Work out the finished part from the listing and answer in its coordinate system (mm). Coordinates: 2 decimals unless noted, no trailing zeros. Write each loop counter-clockwise with the first axis right and the second up, starting at its lowest first coordinate (ties: lowest second). Pieces come first, ordered by that corner, then holes. Notation, with made-up numbers: (39.5, 53.25) - (93.5, 53.25) arc R13 ccw to (93.5, 68.25) - close; hole circle Ø6 at (-7.75, -2). An arc over 180 degrees is marked (long way). One line per item, written item: value.
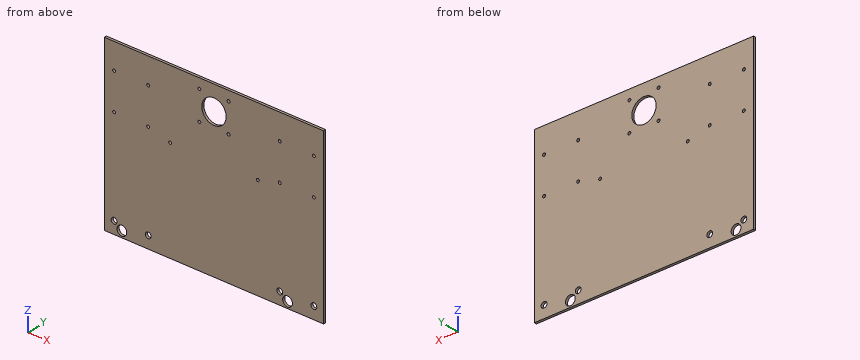
Autodesk Inventor part; units mm, degrees
ref_plane "YZ Plane" through (0, 0, 0) normal (1, 0, 0) x (0, 1, 0)
ref_plane "XZ Plane" through (0, 0, 0) normal (0, 1, 0) x (-1, 0, 0)
ref_plane "XY Plane" through (0, 0, 0) normal (0, 0, 1) x (1, 0, 0)
sketch "Sketch1" plane through (0, 0, 0) normal (0, 1, 0) x (-1, 0, 0)
  line L0 (225, 175) -> (-225, 175)
  line L1 (-225, 175) -> (-225, -175)
  line L2 (-225, -175) -> (225, -175)
  line L3 (225, -175) -> (225, 175)
  line L4 (225, 175) -> (-225, -175) construction
  line L5 (-225, 175) -> (225, -175) construction
  point P0 (0, 0)
  dimension "d0" = 450
  dimension "d1" = 350
extrude "Extrusion1" add sketch "Sketch1" along normal blind 5
sketch "Sketch2" plane through (0, 0, 0) normal (0, -1, 0) x (1, 0, 0)
  line L0 (225, 175) -> (225, -175)
  line L1 (-225, 175) -> (225, 175)
  line L2 (-225, -175) -> (-225, 175)
  line L3 (225, -175) -> (-225, -175)
  line L4 (-198.5, -164) -> (-198.5, -170)
  line L5 (-220, -170) -> (-198.5, -170)
  line L6 (-220, -115) -> (-220, -170)
  line L7 (-220, -115) -> (-120, -115)
  line L8 (-120, -115) -> (-120, -170)
  line L9 (-180, -170) -> (-120, -170)
  line L10 (-180, -170) -> (-180, -159)
  arc A0 (-180, -159) -> (-185, -154) centre (-185, -159) ccw
  line L11 (-185, -154) -> (-188.5, -154)
  arc A1 (-188.5, -154) -> (-198.5, -164) centre (-188.5, -164) ccw
  circle A2 centre (-205, -150) radius 6.1
  circle A3 centre (-135, -150) radius 6.1
  circle A4 centre (-205, 122) radius 3.05
  circle A5 centre (-135, 47) radius 3.05
  circle A6 centre (-135, 122) radius 3.05
  circle A7 centre (-205, 47) radius 3.05
  line L12 (-120, 134.5) -> (-120, 34.5)
  line L13 (-220, 34.5) -> (-120, 34.5)
  line L14 (-220, 134.5) -> (-220, 34.5)
  line L15 (-120, 134.5) -> (-220, 134.5)
  circle A8 centre (30, 95) radius 3.1
  circle A9 centre (30, 155) radius 3.1
  circle A10 centre (-30, 95) radius 3.1
  circle A11 centre (-30, 155) radius 3.1
  circle A12 centre (90, 215) radius 3.1
  circle A13 centre (90, 35) radius 3.1
  circle A14 centre (-90, 215) radius 3.1
  circle A15 centre (-90, 35) radius 3.1
  circle A16 centre (0, 125) radius 25
  line L16 (100, 225) -> (100, 25)
  line L17 (100, 25) -> (-100, 25)
  line L18 (-100, 25) -> (-100, 225)
  line L19 (-100, 225) -> (100, 225)
  circle A17 centre (-205, -150) radius 6
  circle A18 centre (-135, -150) radius 6
  circle A19 centre (-205, 47) radius 3
  circle A20 centre (-205, 122) radius 3
  circle A21 centre (-135, 47) radius 3
  circle A22 centre (-135, 122) radius 3
  circle A23 centre (-90, 35) radius 3
  circle A24 centre (-30, 155) radius 3
  circle A25 centre (-30, 95) radius 3
  point P0 (0, 0)
  dimension "d4" = 12
  dimension "d5" = 12
  dimension "d6" = 6
  dimension "d7" = 6
  dimension "d8" = 6
  dimension "d9" = 6
  dimension "d10" = 6
  dimension "d11" = 6
  dimension "d12" = 6
extrude "Extrusion2" cut sketch "Sketch2" against normal blind 5 contours A17 | A18 | A19 | A20 | A21 | A22 | A23 | A24 | A25
mirror "Mirror1" about plane through (0, 0, 0) normal (1, 0, 0) of "Extrusion2"
sketch "Sketch3" plane through (0, 0, 0) normal (0, -1, 0) x (1, 0, 0)
  circle A0 centre (30, 95) radius 3.1
  circle A1 centre (30, 155) radius 3.1
  circle A2 centre (-30, 95) radius 3.1
  circle A3 centre (-30, 155) radius 3.1
  circle A4 centre (90, 215) radius 3.1
  circle A5 centre (90, 35) radius 3.1
  circle A6 centre (-90, 215) radius 3.1
  circle A7 centre (-90, 35) radius 3.1
  circle A8 centre (0, 125) radius 25
  line L0 (100, 225) -> (100, 25)
  line L1 (100, 25) -> (-100, 25)
  line L2 (-100, 25) -> (-100, 225)
  line L3 (-100, 225) -> (100, 225)
  point P0 (0, 0)
extrude "Extrusion3" cut sketch "Sketch3" against normal blind 5 contours A8
sketch "Sketch6" plane through (0, 5, 0) normal (0, 1, 0) x (1, 0, 0)
  circle A0 centre (0, -125) radius 25
  circle A1 centre (205, -47) radius 3
  circle A2 centre (90, -35) radius 3
  circle A3 centre (30, -95) radius 3
  circle A4 centre (205, -122) radius 3
  circle A5 centre (135, 150) radius 6
  circle A6 centre (135, -122) radius 3
  circle A7 centre (30, -155) radius 3
  circle A8 centre (135, -47) radius 3
  circle A9 centre (205, 150) radius 6
  circle A10 centre (-205, -47) radius 3
  circle A11 centre (-90, -35) radius 3
  circle A12 centre (-30, -95) radius 3
  circle A13 centre (-205, -122) radius 3
  circle A14 centre (-135, 150) radius 6
  circle A15 centre (-135, -122) radius 3
  circle A16 centre (-30, -155) radius 3
  circle A17 centre (-135, -47) radius 3
  circle A18 centre (-205, 150) radius 6
  line L0 (225, -175) -> (225, 175)
  line L1 (225, 175) -> (-225, 175)
  line L2 (-225, 175) -> (-225, -175)
  line L3 (-225, -175) -> (225, -175)
  circle A19 centre (-189, 162) radius 10
  circle A20 centre (151, 162) radius 10
  point P0 (0, 0)
  dimension "d30" = 20
  dimension "d31" = 13
  dimension "d32" = 36
  dimension "d33" = 20
  dimension "d34" = 13
  dimension "d35" = 74
extrude "Extrusion6" cut sketch "Sketch6" against normal blind 5 contours A19 | A20
properties part number "acrylic_upper" material "ABS Plastic"
Item 1: Given pin 1 (5 mm diameter, centred on x = -30, z = 155, fed in from -Y), flat-ended and moving along its own axis, determine where the tip first touches the part or whether it passes through.
Evaluation:
pin 1: passes through
Item 2: Section C-C, the plane y = 3.7 is taken. Give the number of separate pieces and of enclosed holes in the cut face, then the cut area to 3 significant figures.
Evaluation:
separate pieces: 1
enclosed holes: 21
area: 154,000 mm2
Item 3: Section D-D, the plane x = 0 is taken. Determine the outline of the cut face in (y, z).
Evaluation:
outline: (0, -175) - (5, -175) - (5, 100) - (0, 100) - close; (0, 150) - (5, 150) - (5, 175) - (0, 175) - close
Item 4: Section A-A, the plane z = -162 is taken. Determine the outline of the cut face in (x, y), then the cut area to 3 significant figures.
Evaluation:
outline: (-225, 0) - (-199, 0) - (-199, 5) - (-225, 5) - close; (-179, 0) - (141, 0) - (141, 5) - (-179, 5) - close; (161, 0) - (225, 0) - (225, 5) - (161, 5) - close
area: 2,050 mm2
Item 5: Section B-B, the plane x = -189 is taken. Determine the outline of the cut face in (y, z), then the cut area to 3 significant figures.
Evaluation:
outline: (0, -175) - (5, -175) - (5, -172) - (0, -172) - close; (0, -152) - (5, -152) - (5, 175) - (0, 175) - close
area: 1,650 mm2
Item 6: Consider probe 1 along Z at (x, y) = (-30, 3.95); probe 2 along Z at (x, y) = (-135, 3.1); probe 3 along X at (y, z) = (2.15, -162). Determine where each line is inside the solid, lowest interval first.
Evaluation:
probe 1: z = -175 to 92, 98 to 152, 158 to 175
probe 2: z = -175 to -156, -144 to 44, 50 to 119, 125 to 175
probe 3: x = -225 to -199, -179 to 141, 161 to 225
